Geometry: see drawing. Coordinates: mm, zero at the bounding-box minimum. Round coordinates to 2 decimals unless told otherwise and drop trailing zeros. Write each loop counter-clockwise with the first axis right and the second up, starting at its lowest first coordinate (ties: lowest second). Pieces come first, ordered by that corner, then holes. Notation, with made-up numbers: M -8,-36 L 19,-36 A32 cw 19,-2 Z; hole C 78,4 d2. An arc over 180 degrees is marked long. Use one line per item in the form item = value. Start each with the question number.
Item 1: Section query A-A (y = 2.2). Return loops of the section in (x, z).
Item 2: Section query C-C (x = 2.75). Return loops of the section in (y, z), and give its area (3 significant figures).
Item 3: Ray query, probe 1 along X at (y, z) = (2.5, 39); probe 2 along Z at (x, y) = (7.75, 2.85); probe 3 along Z at (x, y) = (14.5, 0.15). Return the intervals inside material, ascending.
Item 4: Section query B-B (z = 55). Return loops of the section in (x, y).
Item 5: Pin query (flat end, axial travel): pin 1 Ø1 at (x, y) = (25, 1) entering from -Z; pin 2 Ø0.9 at (x, y) = (24.5, 1) entering from +Z; pin 3 Ø1.5 at (y, z) = (1, 57) entering from +X. Return the tip coordinate at first contact, or that it passes through.
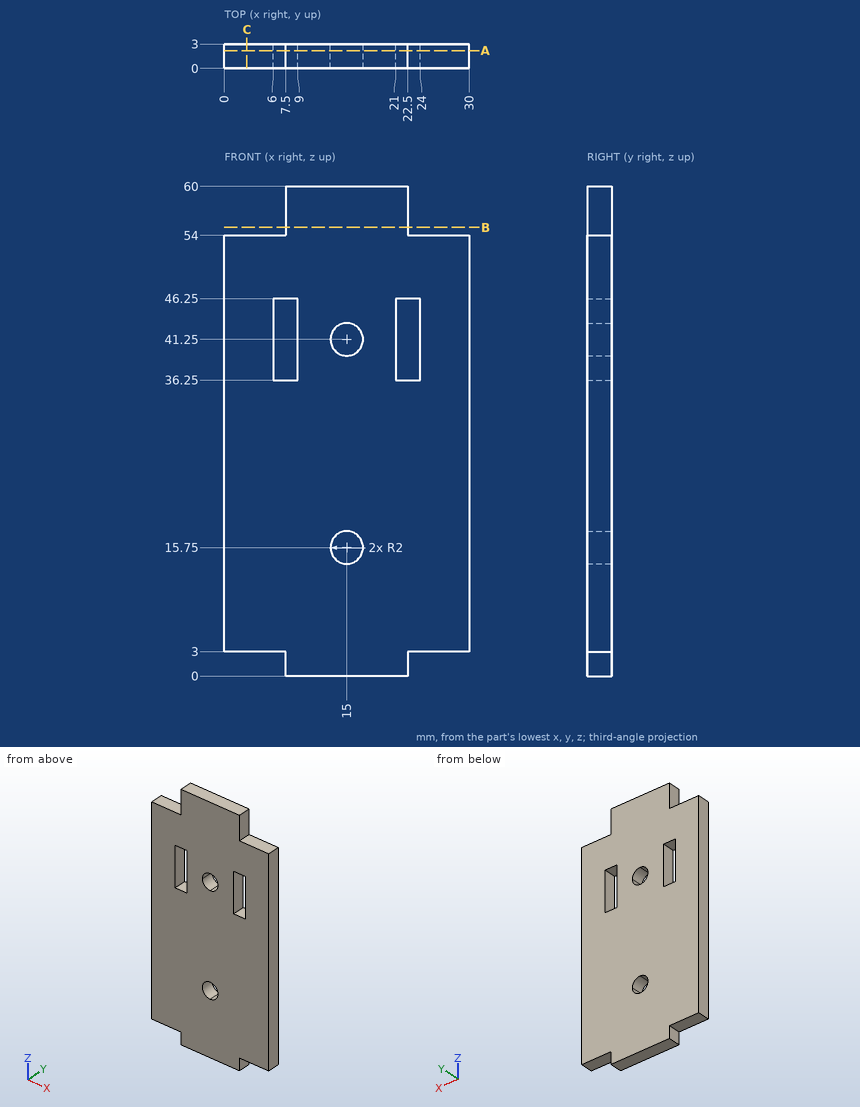
Working result:
q1.outline = M 0,3 L 7.5,3 L 7.5,0 L 22.5,0 L 22.5,3 L 30,3 L 30,54 L 22.5,54 L 22.5,60 L 7.5,60 L 7.5,54 L 0,54 Z; hole M 6,36.25 L 9,36.25 L 9,46.25 L 6,46.25 Z; hole C 15,15.75 d4; hole C 15,41.25 d4; hole M 21,36.25 L 24,36.25 L 24,46.25 L 21,46.25 Z
q2.outline = M 0,3 L 3,3 L 3,54 L 0,54 Z
q2.area = 153 mm²
q3.probe_1 = 0 to 6, 9 to 21, 24 to 30
q3.probe_2 = 0 to 36.25, 46.25 to 60
q3.probe_3 = 0 to 13.81, 17.69 to 39.31, 43.19 to 60
q4.outline = M 7.5,0 L 22.5,0 L 22.5,3 L 7.5,3 Z
q5.pin_1 = 3
q5.pin_2 = 54
q5.pin_3 = 22.5
